```python
from build123d import *

# Parameters (mm, degrees)
SKETCH1_W           = 48.26
SKETCH1_H           = 17.78
BOSS_EXTRUDE1_DEPTH = 15.24
CUT_EXTRUDE1_DEPTH  = 7.62
CUT_EXTRUDE2_DEPTH  = 54.641528688
SKETCH5_W           = 15.24
SKETCH5_H           = 10.16
BOSS_EXTRUDE2_DEPTH = 3.75
CUT_EXTRUDE5_DEPTH  = 7.62
CUT_EXTRUDE7_DEPTH  = 7.62


with BuildPart() as part:
    # Sketch1 → Boss-Extrude1 (new body)
    with BuildSketch(Plane.XY):
        with Locations((24.13, 8.89)):
            Rectangle(SKETCH1_W, SKETCH1_H)
    extrude(amount=-BOSS_EXTRUDE1_DEPTH)

    # Sketch3 → Cut-Extrude1 (cut)
    with BuildSketch(Plane(origin=(0, 17.78, 0), x_dir=(1, 0, 0), z_dir=(0, 1, 0))):
        Polygon((48.26, 15.24), (40.64, 7.62), (48.26, 0), align=None)
    extrude(amount=-CUT_EXTRUDE1_DEPTH, mode=Mode.SUBTRACT)

    # Sketch4 → Cut-Extrude2 (cut, through all)
    with BuildSketch(Plane(origin=(0, 17.78, 0), x_dir=(1, 0, 0), z_dir=(0, 1, 0))):
        with BuildLine():
            Line((34.83, 5.62), (27.21, 5.62))
            ThreePointArc((27.21, 5.62), (25.21, 7.62), (27.21, 9.62))
            Line((27.21, 9.62), (34.83, 9.62))
            ThreePointArc((34.83, 9.62), (36.83, 7.62), (34.83, 5.62))
        make_face()
        with BuildLine():
            Line((18.13, 5.62), (10.51, 5.62))
            ThreePointArc((10.51, 5.62), (8.51, 7.62), (10.51, 9.62))
            Line((10.51, 9.62), (18.13, 9.62))
            ThreePointArc((18.13, 9.62), (20.13, 7.62), (18.13, 5.62))
        make_face()
    extrude(amount=-CUT_EXTRUDE2_DEPTH, mode=Mode.SUBTRACT)

    # Sketch5 → Boss-Extrude2 (add)
    with BuildSketch(Plane(origin=(48.26, 0, 0), x_dir=(0, 0, -1), z_dir=(1, 0, 0))):
        with Locations((7.62, 5.08)):
            Rectangle(SKETCH5_W, SKETCH5_H)
    extrude(amount=BOSS_EXTRUDE2_DEPTH)

    # Sketch6 → Cut-Extrude5 (cut)
    with BuildSketch(Plane(origin=(0, 17.78, 0), x_dir=(1, 0, 0), z_dir=(0, 1, 0))):
        Polygon((48.26, 0), (46.76, 0), (46.76, 1.5), align=None)
    extrude(amount=-CUT_EXTRUDE5_DEPTH, mode=Mode.SUBTRACT)

    # Sketch7 → Cut-Extrude7 (cut)
    with BuildSketch(Plane(origin=(0, 17.78, 0), x_dir=(1, 0, 0), z_dir=(0, 1, 0))):
        Polygon((48.26, 15.24), (46.76, 15.24), (46.76, 13.74), align=None)
    extrude(amount=-CUT_EXTRUDE7_DEPTH, mode=Mode.SUBTRACT)


solid = part.part
```
The listing builds one solid part. Answer for the finished solid, in the listing's coordinates (mm). A direction names the side the tool comes from. Round coordinates to 2 decimals unless told otherwise and drop trailing zeros. Write each loop counter-clockwise with the first axis right and the second up, starting at its lowest first coordinate (ties: lowest second). Pieces come first, ordered by that corner, then holes. Notation, with made-up numbers: (-8, 18) -> (5, 18) arc R24 cw to (5, 44) -> close; hole circle Ø2 at (32.25, 1.5). An arc over 180 degrees is marked (long way). Write item = value, one per line.
1) Section C-C on z = -7 is taken. Write down the section's boundary in (x, y), plus the area to 3 significant figures.
Check values:
outline = (0, 0) -> (8.61, 0) -> (8.61, 17.78) -> (0, 17.78) -> close; (20.03, 0) -> (25.31, 0) -> (25.31, 17.78) -> (20.03, 17.78) -> close; (36.73, 0) -> (52.01, 0) -> (52.01, 10.16) -> (41.26, 10.16) -> (41.26, 17.78) -> (36.73, 17.78) -> close
area = 437 mm²
2) Given pin 1 (0.8 mm diameter, centred on y = 12.5, z = -0.5, fed in from +X), flat-ended and moving along its own axis, determine where the tip first touches the part or whether it passes through.
Check values:
pin_1 = 46.76
3) Which of the six approach directions +Z, -Z, +X, -X, +Y, -Y give full straight-line access (tool end or side, diameter ignored) to faces 5 (the flat face through (46.76, 14, -1)), 6 (the flat face through (48, 10.16, -8)), 7 (the flat face through (25.6, 0, -9.2)), 8 (the flat face through (14, 9, -9.62))?
Check values:
face_5 = +Z, -Z, +X, +Y
face_6 = +X, +Y
face_7 = +Z, -Z, +X, -X, -Y
face_8 = +Y, -Y
4) Section A-A on x = 28.5 is taken. Write down the section's boundary in (y, z).
Check values:
outline = (0, -15.24) -> (17.78, -15.24) -> (17.78, -9.62) -> (0, -9.62) -> close; (0, -5.62) -> (17.78, -5.62) -> (17.78, 0) -> (0, 0) -> close
5) Section B-B on y = 13.25 is taken. Write down the section's boundary in (x, z).
Check values:
outline = (0, -15.24) -> (46.76, -15.24) -> (46.76, -13.74) -> (40.64, -7.62) -> (46.76, -1.5) -> (46.76, 0) -> (0, 0) -> close; hole (10.51, -9.62) -> (18.13, -9.62) arc R2 ccw to (18.13, -5.62) -> (10.51, -5.62) arc R2 ccw to start; hole (27.21, -9.62) -> (34.83, -9.62) arc R2 ccw to (34.83, -5.62) -> (27.21, -5.62) arc R2 ccw to start
6) Section D-D on x = 19 is taken. Write down the section's boundary in (y, z).
Check values:
outline = (0, -15.24) -> (17.78, -15.24) -> (17.78, -9.42) -> (0, -9.42) -> close; (0, -5.82) -> (17.78, -5.82) -> (17.78, 0) -> (0, 0) -> close
7) For a pull along Z with two mould halves and no side action, classify faces 1 (the cylindrical face through (20.13, 9.01, -7.66)), 2 (the flat face through (46.76, 14, -15)), 3 (the flat face through (26, 9, -15.24)), 4 (the flat face through (26, 9, 0)) as released by +Z, released by -Z, zero draft, split by the parting line, or undercut.
Check values:
face_1 = undercut
face_2 = zero draft
face_3 = released by -Z
face_4 = released by +Z
8) Straight lines are drawn through the part: line 1 along Z through (x, y) = (30.5, 13.25); line 2 along X through (y, z) = (4.5, -7.25); line 3 along X through (y, z) = (9.5, -8.5). For each, find the intervals that lie inside material, in ascending order. Write a range as [from, to].
Check values:
line_1 = [-15.24, -9.62], [-5.62, 0]
line_2 = [0, 8.54], [20.1, 25.24], [36.8, 52.01]
line_3 = [0, 8.71], [19.93, 25.41], [36.63, 52.01]
